Can you work these out from the model? Positions are in its coordinate system, mm. Face numbers are marked on the shaded views. Round coordinates to 2 decimals unless told otherwise and drop trailing zeros. Loops run counter-clockwise (first coordinate to the right, second up) from the corner with the lowest first, then second, coordinate; pieces in that order, holes last. Notation, with made-up numbers: (-11.5, -2.75) -> (16.5, -2.75) arc R24 cw to (16.5, 10.25) -> close; hole circle Ø11 at (-29, -29.5). An arc over 180 degrees is marked (long way). Write item = value, one per line.
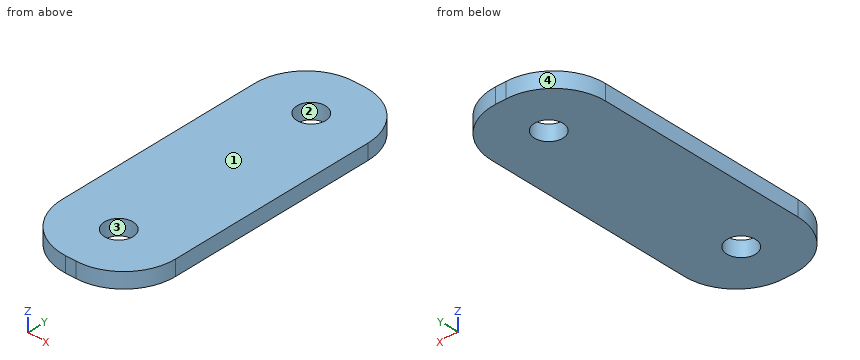
Autodesk Inventor part; units mm, degrees
ref_plane "YZ Plane" through (0, 0, 0) normal (1, 0, 0) x (0, 1, 0)
ref_plane "XZ Plane" through (0, 0, 0) normal (0, 1, 0) x (-1, 0, 0)
ref_plane "XY Plane" through (0, 0, 0) normal (0, 0, 1) x (1, 0, 0)
sketch "Skizze1" plane through (0, 0, 0) normal (0, 0, 1) x (1, 0, 0)
  line L0 (-15.4, 0) -> (15.4, 0)
  line L1 (0, -42) -> (0, 42)
  line L2 (11, -30) -> (-11, -30)
  line L3 (-11, -30) -> (-11, 30)
  line L4 (-11, 30) -> (11, 30)
  line L5 (11, 30) -> (11, -30)
  line L6 (11, -30) -> (-11, 30) construction
  line L7 (-11, -30) -> (11, 30) construction
  point P0 (0, 0)
  dimension "d0" = 60
  dimension "d1" = 22
extrude "Extrusion1" add sketch "Skizze1" along normal blind 3
sketch "Skizze2" plane through (0, 0, 3) normal (0, 0, 1) x (1, 0, 0)
  line L0 (11, 30) -> (-11, 30)
  line L1 (-11, 30) -> (-11, -30)
  line L2 (-11, -30) -> (11, -30)
  line L3 (11, -30) -> (11, 30)
  line L4 (-17.5, 0) -> (17.5, 0)
  line L5 (0, -42) -> (0, 42)
  line L6 (3.1579, -20) -> (-3.1579, -20)
  line L7 (-3.1579, -20) -> (-3.1579, 20)
  line L8 (-3.1579, 20) -> (3.1579, 20)
  line L9 (3.1579, 20) -> (3.1579, -20)
  line L10 (3.1579, -20) -> (-3.1579, 20) construction
  line L11 (-3.1579, -20) -> (3.1579, 20) construction
  point P0 (0, 0)
  point P1 (0, 20)
  point P2 (0, -20)
  dimension "d4" = 40
hole "Bohrung1" at (0, 20, 3) at (0, -20, 3) direction (0, 0, -1) diameter 5.5 end through all
fillet "Rundung1" radius 10 4 edges at (-11, 30, 1.5) (11, 30, 1.5) (11, -30, 1.5) (-11, -30, 1.5)
sketch "Skizze3" plane through (0, 0, 3) normal (0, 0, 1) x (1, 0, 0)
  point P0 (0, 0)
properties part number "24_0497_0012" material "PMMA-Kunststoff"
1. I need wall thicknesses on line 1 (Y direction, x = 0, z = 1.2); line 2 (X direction, y = -20, z = 0.95); line 3 (Y direction, x = -1.75, z = 1.9). Which ranges of each line are inside material? Lowest first, please. Write a range as [from, to].
Entries:
line_1 = [-30, -22.75], [-17.25, 17.25], [22.75, 30]
line_2 = [-11, -2.75], [2.75, 11]
line_3 = [-29.97, -22.12], [-17.88, 17.88], [22.12, 29.97]
2. Suppose I cut it at A-A, the plane x = 0. List the corners of the cut face in (y, z) for me.
Entries:
outline = (-30, 0) -> (-22.75, 0) -> (-22.75, 3) -> (-30, 3) -> close; (-17.25, 0) -> (17.25, 0) -> (17.25, 3) -> (-17.25, 3) -> close; (22.75, 0) -> (30, 0) -> (30, 3) -> (22.75, 3) -> close
3. We'd pull the mould along X, two halves only. Please class the marked faces 1, 2, 3 and 4: released by +X, released by -X, zero draft, split by the parting line, or undercut.
Entries:
face_1 = zero draft
face_2 = undercut
face_3 = undercut
face_4 = released by -X
4. Suppose I cut it at D-D, the plane x = 4.25. List the corners of the cut face in (y, z) for me.
Entries:
outline = (-29.46, 0) -> (29.46, 0) -> (29.46, 3) -> (-29.46, 3) -> close
5. Suppose I cut it at C-C, the plane x = 7. List the corners of the cut face in (y, z) for me.
Entries:
outline = (-28, 0) -> (28, 0) -> (28, 3) -> (-28, 3) -> close
6. I'm going to push a flat-ended pin straight in: pin 1 (1 mm diameter, centred on x = -5, z = 2.5, fed in from +Y). Where does the tip first touch, or does it pass through?
Entries:
pin_1 = 29.37
7. Suppose I cut it at B-B, the plane z = 1.95. List the corners of the cut face in (x, y) for me.
Entries:
outline = (-11, -20) arc R10 ccw to (-1, -30) -> (1, -30) arc R10 ccw to (11, -20) -> (11, 20) arc R10 ccw to (1, 30) -> (-1, 30) arc R10 ccw to (-11, 20) -> close; hole circle Ø5.5 at (0, -20); hole circle Ø5.5 at (0, 20)
